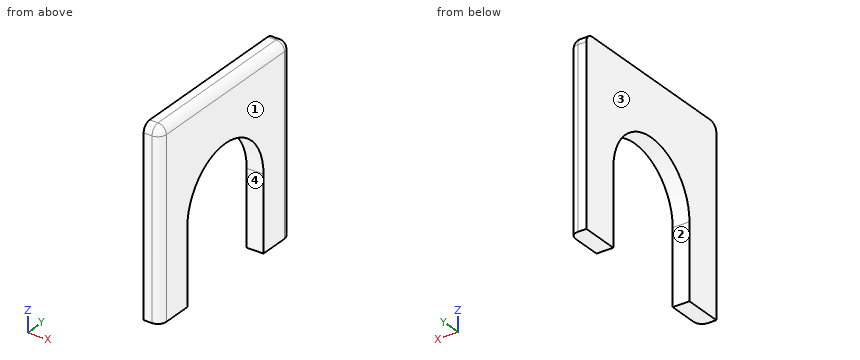
```python
from build123d import *

# Parameters (mm, degrees)
F0_W     = 279.4
F0_H     = 279.4
F1_DEPTH = 25.4
F3_DEPTH = 25.4
F4_R     = 12.7
F5_R     = 12.7


with BuildPart() as f1:
    # F0 (on Right) → F1 (new body)
    with BuildSketch(Plane.YZ):
        with Locations((139.7, 139.7)):
            Rectangle(F0_W, F0_H)
    extrude(amount=F1_DEPTH)

    # F2 (on face) → F3 (cut)
    with BuildSketch(Plane.YZ.offset(25.4)):
        with BuildLine():
            Line((221.641318, -113.265621), (221.641318, 113.265621))
            ThreePointArc((221.641318, 113.265621), (139.7, 195.20694), (57.758682, 113.265621))
            Line((57.758682, 113.265621), (57.758682, -113.265621))
            Line((57.758682, -113.265621), (221.641318, -113.265621))
        make_face()
    extrude(amount=-F3_DEPTH, mode=Mode.SUBTRACT)

    # F4
    f4_edges = [f1.edges().sort_by_distance(p)[0] for p in [
        (12.7, 0, 279.4),
        (12.7, 279.4, 279.4),
    ]]
    fillet(f4_edges, radius=F4_R)

    # F5
    f5_edges = [f1.edges().sort_by_distance(p)[0] for p in [
        (25.4, 139.7, 279.4),
    ]]
    fillet(f5_edges, radius=F5_R)


solid = f1.part
```
Input: part model. Units: mm. Frame: model coordinates. Face numbers are marked on the shaded views. A direction names the side the tool comes from. Round coordinates to 2 decimals unless told otherwise and drop trailing zeros. Order: outer loops, then holes, each group sorted by start corner. A loop starts at its lowest first (then second) coordinate and runs counter-clockwise, first axis right, second up. Notation, with made-up numbers: (-32.75, -9.75) - (-22.75, -9.75) arc R23 ccw to (-22.75, 26.25) - close; hole circle Ø10 at (85.25, 8.5). An arc over 180 degrees is marked (long way). Answer in a Markdown table with one row per item.
Item 1: Mould query, pull axis Y, two halves, no side actions, for the marked faces 3 and 4. Classes: released by +Y, released by -Y, zero draft, split by the parting line, or undercut.
Model answer:
| item | result |
|---|---|
| face 3 | zero draft |
| face 4 | undercut |
Item 2: Pin query (flat end, axial travel): pin 1 (1 mm diameter, centred on y = 52, z = 213, fed in from -X); pin 2 (1 mm diameter, centred on x = 14.5, z = 197.5, fed in from -Y); pin 3 (4 mm diameter, centred on x = 15, y = 38.5, fed in from +Z). Return the tip coordinate at first contact, or that it passes through.
Model answer:
| item | result |
|---|---|
| pin 1 | stops at x = 0 |
| pin 2 | stops at y = 0.07 |
| pin 3 | stops at z = 279.4 |
Item 3: Section query B-B (x = 4.75). Return the cut outline in (y, z), then the cut area to 3 significant figures.
Model answer:
| item | result |
|---|---|
| outline | (0, 0) - (57.76, 0) - (57.76, 113.27) arc R81.94 cw to (221.64, 113.27) - (221.64, 0) - (279.4, 0) - (279.4, 266.7) arc R12.7 ccw to (266.7, 279.4) - (12.7, 279.4) arc R12.7 ccw to (0, 266.7) - close |
| area | 48,900 mm² |
Item 4: Section query C-C (y = 139.7). Return the cut outline in (x, z).
Model answer:
| item | result |
|---|---|
| outline | (0, 195.21) - (25.4, 195.21) - (25.4, 266.7) arc R12.7 ccw to (12.7, 279.4) - (0, 279.4) - close |
Item 5: Line query: line 1 (Y direction, x = 1, z = 29); line 2 (Z direction, x = 13.75, y = 238.5); line 3 (Y direction, x = 12.25, z = 135). Output: solid intervals per line, ascending.
Model answer:
| item | result |
|---|---|
| line 1 | y = 0 to 57.76, 221.64 to 279.4 |
| line 2 | z = 0 to 279.36 |
| line 3 | y = 0 to 60.69, 218.71 to 279.4 |
Item 6: Section query A-A (z = 42). Return the cut outline in (x, y).
Model answer:
| item | result |
|---|---|
| outline | (0, 0) - (12.7, 0) arc R12.7 ccw to (25.4, 12.7) - (25.4, 57.76) - (0, 57.76) - close; (0, 221.64) - (25.4, 221.64) - (25.4, 266.7) arc R12.7 ccw to (12.7, 279.4) - (0, 279.4) - close |
Item 7: Section query D-D (z = 170). Return the cut outline in (x, y).
Model answer:
| item | result |
|---|---|
| outline | (0, 0) - (12.7, 0) arc R12.7 ccw to (25.4, 12.7) - (25.4, 80.58) - (0, 80.58) - close; (0, 198.82) - (25.4, 198.82) - (25.4, 266.7) arc R12.7 ccw to (12.7, 279.4) - (0, 279.4) - close |
Item 8: Reachability of the marked faces 1 and 2 from +Z, -Z, +X, -X, +Y, -Y: full face, straight path, thin tool, end or side. Return the list, or none.
Model answer:
| item | result |
|---|---|
| face 1 | +Z, -Z, +X, +Y, -Y |
| face 2 | -Z, +X, -X |
